Build history of the part. All positions in model axes, mm. A direction names the side the tool comes from. Round coordinates to 2 decimals unless told otherwise and drop trailing zeros. Write each loop counter-clockwise with the first axis right and the second up, starting at its lowest first coordinate (ties: lowest second). Pieces come first, ordered by that corner, then holes.
Item 1: Band-saw the part on A-A, the plane x = 0. Write the cut outline in (y, z), then the cut area to 3 significant figures.
Item 2: Mould opens along Y. For faces 1 (the flat face through (-1, 251, -50)), 2 (the flat face through (-1, 1, 175)), 3 (the cylindrical face through (1.08, 298.99, -25.35)) say: +Y half, -Y half, draft (parallel to the pull), parting line (faces both ways), or undercut.
Item 3: Wall check: probe 1 along Z at (x, y) = (35.5, 58); probe 2 along Y at (x, z) = (0, -55.25); probe 3 along Z at (x, y) = (24, 34). Give the ranges that are in metal, low to high.
Item 4: Drop flat-ended pins along their axis: pin 1 Ø1 at (x, z) = (1, 31.5) entering from -Y; pin 2 Ø8 at (x, z) = (-13, 56.5) entering from +Y; pin 3 Ø8 at (x, y) = (-29, 247.5) entering from +Z. Give the stop position or say it passes through.
Item 5: Band-saw the part on C-C, the plane z = 6. Write the cut outline in (x, y), then the cut area to 3 significant figures.
Item 6: Band-saw the part on D-D, the plane x = 15.5. Write the cut outline in (y, z).
Item 7: 3-axis set-ups, long thin cutter, end or side, ignore diameter. For faces 4 (the cylindrical face through (5.858, 294.617, -62.325)), 5 (the flat face through (49, 123, -25)): which of +Z, -Z, +X, -X, +Y, -Y reach the whole face in a straight line?
Item 8: Band-saw the part on B-B, the plane y = 229.5. Write the cut outline in (x, z), then the cut area to 3 significant figures.
```python
from build123d import *

# Parameters (mm, degrees)
SKETCH1_R           = 49
BOSS_EXTRUDE1_DEPTH = 175
BOSS_EXTRUDE2_START = 50
BOSS_EXTRUDE2_DEPTH = 50
SKETCH3_R           = 47.5
SKETCH3_R_2         = 45
BOSS_EXTRUDE3_DEPTH = 25


with BuildPart() as part:
    # Sketch1 → Boss-Extrude1 (new body)
    with BuildSketch(Plane.XY):
        Circle(SKETCH1_R)
    extrude(amount=BOSS_EXTRUDE1_DEPTH)

    # Sketch2 → Boss-Extrude2 (add)
    with BuildSketch(Plane(origin=(0, 0, 0), x_dir=(-1, 0, 0), z_dir=(0, 0, -1)).offset(BOSS_EXTRUDE2_START)):
        with BuildLine():
            Line((-49, 0), (-49, 250))
            ThreePointArc((-49, 250), (0, 299), (49, 250))
            Line((49, 250), (49, 0))
            ThreePointArc((49, 0), (0, -49), (-49, 0))
        make_face()
    extrude(amount=-BOSS_EXTRUDE2_DEPTH)

    # Sketch3 → Boss-Extrude3 (add)
    with BuildSketch(Plane(origin=(0, 0, -50), x_dir=(-1, 0, 0), z_dir=(0, 0, -1))):
        with Locations((0, 250)):
            Circle(SKETCH3_R)
        with Locations((0, 250)):
            Circle(SKETCH3_R_2, mode=Mode.SUBTRACT)
    extrude(amount=BOSS_EXTRUDE3_DEPTH)


solid = part.part
```
Results:
1. outline: (-49, -50) - (202.5, -50) - (202.5, -75) - (205, -75) - (205, -50) - (295, -50) - (295, -75) - (297.5, -75) - (297.5, -50) - (299, -50) - (299, 0) - (49, 0) - (49, 175) - (-49, 175) - close
1. area: 34,700 mm2
2. face 1: undercut
2. face 2: draft
2. face 3: +Y half
3. probe 1: z = -50 to 0
3. probe 2: y = 202.5 to 205, 295 to 297.5
3. probe 3: z = -50 to 175
4. pin 1: stops at y = -49
4. pin 2: stops at y = 48.17
4. pin 3: stops at z = 0
5. outline: circle Ø98 at (0, 0)
5. area: 7,540 mm2
6. outline: (-46.48, -50) - (205.1, -50) - (205.1, -75) - (207.75, -75) - (207.75, -50) - (292.25, -50) - (292.25, -75) - (294.9, -75) - (294.9, -50) - (296.48, -50) - (296.48, 0) - (46.48, 0) - (46.48, 175) - (-46.48, 175) - close
7. face 4: -Z
7. face 5: +Z, -Z, +X, +Y, -Y
8. outline: (-49, -50) - (-42.85, -50) - (-42.85, -75) - (-40.06, -75) - (-40.06, -50) - (40.06, -50) - (40.06, -75) - (42.85, -75) - (42.85, -50) - (49, -50) - (49, 0) - (-49, 0) - close
8. area: 5,040 mm2
